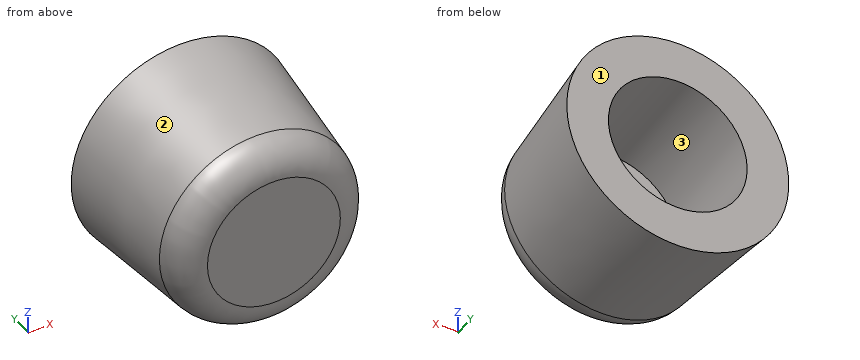
```python
from build123d import *

# Parameters (mm, degrees)
F0_R     = 17.78
F2_R     = 15.24
F4_R     = 5.08
F5_R     = 11.1125
F6_DEPTH = 19.05


with BuildPart() as f3:
    # F0 (on Front) → F3 section 0
    with BuildSketch(Plane.XZ):
        Circle(F0_R)
    # F2 (on offset) → F3 section 1
    with BuildSketch(Plane.XZ.offset(25.4)):
        Circle(F2_R)
    loft()

    # F4
    f4_edges = [f3.edges().sort_by_distance(p)[0] for p in [
        (-15.24, -25.4, 0),
    ]]
    fillet(f4_edges, radius=F4_R)

    # F5 (on face) → F6 (cut)
    with BuildSketch(Plane(origin=(0, 0, 0), x_dir=(-1, 0, 0), z_dir=(0, 1, 0))):
        Circle(F5_R)
    extrude(amount=-F6_DEPTH, mode=Mode.SUBTRACT)


solid = f3.part
```
Could you check a few things on this model? Use its own coordinates, in mm. Face numbers are marked on the shaded views. Round coordinates to 2 decimals unless told otherwise and drop trailing zeros. Loops run counter-clockwise (first coordinate to the right, second up) from the corner with the lowest first, then second, coordinate; pieces in that order, holes last. Notation, with made-up numbers: M -20.75,12.5 L 12.25,12.5 A11 ccw 12.25,29.5 Z; hole C 5.5,51 d4. An arc over 180 degrees is marked long. Write item = value, one per line.
1. Will these pins go through, and if not, where does the flat tip stop? P1, Ø4, axis at y = -18.5, z = 2.5, coming from the -X side; P2, Ø3, axis at x = -6, z = -6, coming from the +Y side; P3, Ø5, axis at x = 13.5, y = -15, coming from the -Z side.
Results below:
P1 = -16.04
P2 = -19.05
P3 = -12.03
2. I want a section at A-A, the plane x = 0. Write out the boundary of the cut face in (y, z).
Results below:
outline = M -25.4,-10.64 A5.08 ccw -20.83,-15.7 L 0,-17.78 L 0,-11.11 L -19.05,-11.11 L -19.05,11.11 L 0,11.11 L 0,17.78 L -20.83,15.7 A5.08 ccw -25.4,10.64 Z
3. I need wall thicknesses on probe 1 along Y at (x, z) = (1.5, 3); probe 2 along X at (y, z) = (-3.25, 1); probe 3 along Z at (x, y) = (0, -4.75) (1 decimal). Which ranges of each line are inside material? Lowest first, please.
Results below:
probe_1 = -25.4 to -19.05
probe_2 = -17.43 to -11.07, 11.07 to 17.43
probe_3 = -17.3 to -11.1, 11.1 to 17.3
4. I want a section at D-D, the plane y = -22.5. Write out the boundary of the cut face in (x, z), and give its area (3 significant figures).
Results below:
outline = C 0,0 d30.46
area = 729 mm²
5. I want a section at C-C, the plane y = -17.25. Write out the boundary of the cut face in (x, z) (1 decimal), and give its area (3 significant figures).
Results below:
outline = C 0,0 d32.1; hole C 0,0 d22.2
area = 422 mm²
6. I want a section at B-B, the plane y = -1.5. Write out the boundary of the cut face in (x, z) (1 decimal).
Results below:
outline = C 0,0 d35.3; hole C 0,0 d22.2
7. Thinking about a two-plate mould opening in Z: for the marked faces 1, 2 and 3, which applies, +Z half, -Z half, draft (parallel to the pull), parting line (faces both ways), or undercut?
Results below:
face_1 = draft
face_2 = parting line
face_3 = undercut
